Verification items for the finished model (mm, model axes). Round coordinates to 2 decimals unless told otherwise and drop trailing zeros. Write each loop counter-clockwise with the first axis right and the second up, starting at its lowest first coordinate (ties: lowest second). Pieces come first, ordered by that corner, then holes. Notation, with made-up numbers: (81.25, -31) - (127.25, -31) arc R35 ccw to (127.25, 5) - close; hole circle Ø7 at (19, 67). An arc over 180 degrees is marked (long way). Answer as a JSON object with one key per item and string values. Group by question number.
1) Mould release check, pull along X, two halves, no side actions. Record for faces 1 (the flat face through (-4, 4, 0)), 2 (the cylindrical face through (-33.037, -275.776, 39.889)), 3 (the cylindrical face through (-4.96, 240.976, 12.522)): +X half, -X half, draft (parallel to the pull), parting line (faces both ways), or undercut.
2) Section check B-B (z = 14). Enter the section's corners in (x, y).
3) Thickness scan on line 1 (Y direction, x = 0, z = 19.5); line 2 (Z direction, x = -231.5, y = -61.5); line 3 (Y direction, x = 82, z = 39). Record the ranges inside material, lowest first.
4) Go/stop test with flat-tipped pins: pin 1 Ø1.5 at (x, z) = (-42.5, 17) entering from +Y; pin 2 Ø1.5 at (x, z) = (-97, 41.5) entering from +Y; pin 3 Ø2 at (y, z) = (-38, 12.5) entering from -X. Record where each tip stops, or that it passes through.
5) Section check A-A (x = 0). Enter the section's corners in (y, z).
```python
from build123d import *

# Parameters (mm, degrees)
SKETCH1_R           = 304.8
SKETCH1_R_2         = 101.6
SKETCH1_R_3         = 38.1
BOSS_EXTRUDE1_DEPTH = 25.4
SKETCH2_R           = 152.4
SKETCH2_R_2         = 101.6
BOSS_EXTRUDE2_DEPTH = 25.4
FILLET1_R           = 2.54
FILLET2_R           = 6.35


with BuildPart() as part:
    # Sketch1 → Boss-Extrude1 (new body)
    with BuildSketch(Plane.XY):
        Circle(SKETCH1_R)
        with Locations((0, -127)):
            Circle(SKETCH1_R_2, mode=Mode.SUBTRACT)
        with Locations((0, 203.2)):
            Circle(SKETCH1_R_3, mode=Mode.SUBTRACT)
    extrude(amount=BOSS_EXTRUDE1_DEPTH)

    # Sketch2 → Boss-Extrude2 (add)
    with BuildSketch(Plane.XY.offset(25.4)):
        with Locations((0, -127)):
            Circle(SKETCH2_R)
        with Locations((0, -127)):
            Circle(SKETCH2_R_2, mode=Mode.SUBTRACT)
    extrude(amount=BOSS_EXTRUDE2_DEPTH)

    # Fillet1
    fillet1_edges = [part.edges().sort_by_distance(p)[0] for p in [
        (-152.4, -127, 50.8),
        (-304.8, 0, 0),
        (-304.8, 0, 25.4),
    ]]
    fillet(fillet1_edges, radius=FILLET1_R)

    # Fillet2
    fillet2_edges = [part.edges().sort_by_distance(p)[0] for p in [
        (-152.4, -127, 25.4),
    ]]
    fillet(fillet2_edges, radius=FILLET2_R)


solid = part.part
```
Returned:
{
 "1": {"face 1": "draft", "face 2": "parting line", "face 3": "undercut"},
 "2": {"outline": "circle Ø609.6 at (0, 0); hole circle Ø203.2 at (0, -127); hole circle Ø76.2 at (0, 203.2)"},
 "3": {"line 1": "-304.8 to -228.6, -25.4 to 165.1, 241.3 to 304.8", "line 2": "0 to 25.4", "line 3": "-255.46 to -186.99, -67.01 to 1.46"},
 "4": {"pin 1": "y = 301.93", "pin 2": "y = -8.84", "pin 3": "x = -302.55"},
 "5": {"outline": "(-304.8, 2.54) arc R2.54 ccw to (-302.26, 0) - (-228.6, 0) - (-228.6, 50.8) - (-276.86, 50.8) arc R2.54 ccw to (-279.4, 48.26) - (-279.4, 31.75) arc R6.35 cw to (-285.75, 25.4) - (-302.26, 25.4) arc R2.54 ccw to (-304.8, 22.86) - close; (-25.4, 0) - (165.1, 0) - (165.1, 25.4) - (31.75, 25.4) arc R6.35 cw to (25.4, 31.75) - (25.4, 48.26) arc R2.54 ccw to (22.86, 50.8) - (-25.4, 50.8) - close; (241.3, 0) - (302.26, 0) arc R2.54 ccw to (304.8, 2.54) - (304.8, 22.86) arc R2.54 ccw to (302.26, 25.4) - (241.3, 25.4) - close"}
}
